Can you work these out from the model? Positions are in its coordinate system, mm. Coordinates: 2 decimals unless noted, no trailing zeros. Order: outer loops, then holes, each group sorted by start corner. A loop starts at its lowest first (then second) coordinate and runs counter-clockwise, first axis right, second up. Notation, with made-up numbers: (30.25, 10) -> (52.25, 10) arc R24 ccw to (52.25, 24) -> close; hole circle Ø3 at (89, -18). An arc over 180 degrees is marked (long way). Answer as a JSON object with one key per item and string values. Group by question number.
(1) I want a section at A-A, the plane x = -56. List the corners of the cut face in (y, z) for me, plus the area to 3 significant figures.
(2) If we mould it in two halves opening along X, with no side actions, what happens to faces 1 (the cylindrical face through (-65.287, 3.219, 9.248)), 2 (the flat face through (-1, 6.35, 0)), 3 (the cylindrical face through (-58.747, 3.131, -0.121))? For each: pulls with the +X half, pulls with the -X half, needs draft (parallel to the pull), parting line crosses it, or undercut.
(3) I want a section at B-B, the plane z = 0. List the corners of the cut face in (x, y) for me.
(4) I need wall thicknesses on line 1 (X direction, y = 1.75, z = 0); line 2 (Z direction, x = -56, y = 1.75); line 3 (X direction, y = 2.5, z = -2). Which ranges of each line are inside material? Lowest first, please.
(5) I want a section at C-C, the plane y = 4.75. List the corners of the cut face in (x, z) for me, plus the area to 3 significant figures.
from build123d import *

# Parameters (mm, degrees)
SKETCH1_W           = 132
SKETCH1_H           = 20
SKETCH1_R           = 2.75
BOSS_EXTRUDE1_DEPTH = 6.35
FILLET1_R           = 2.5


with BuildPart() as part:
    # Sketch1 → Boss-Extrude1 (new body)
    with BuildSketch(Plane(origin=(0, 0, 0), x_dir=(1, 0, 0), z_dir=(0, 1, 0))):
        Rectangle(SKETCH1_W, SKETCH1_H)
        with Locations((-56, 0)):
            Circle(SKETCH1_R, mode=Mode.SUBTRACT)
        with Locations((56, 0)):
            Circle(SKETCH1_R, mode=Mode.SUBTRACT)
    extrude(amount=BOSS_EXTRUDE1_DEPTH)

    # Fillet1
    fillet1_edges = [part.edges().sort_by_distance(p)[0] for p in [
        (-66, 3.175, -10),
        (66, 3.175, -10),
        (66, 3.175, 10),
        (-66, 3.175, 10),
    ]]
    fillet(fillet1_edges, radius=FILLET1_R)


solid = part.part
Computed values:
{
 "1": {"outline": "(0, -10) -> (6.35, -10) -> (6.35, -2.75) -> (0, -2.75) -> close; (0, 2.75) -> (6.35, 2.75) -> (6.35, 10) -> (0, 10) -> close", "area": "92.1 mm2"},
 "2": {"face 1": "pulls with the -X half", "face 2": "needs draft", "face 3": "undercut"},
 "3": {"outline": "(-66, 0) -> (-58.75, 0) -> (-58.75, 6.35) -> (-66, 6.35) -> close; (-53.25, 0) -> (53.25, 0) -> (53.25, 6.35) -> (-53.25, 6.35) -> close; (58.75, 0) -> (66, 0) -> (66, 6.35) -> (58.75, 6.35) -> close"},
 "4": {"line 1": "x = -66 to -58.75, -53.25 to 53.25, 58.75 to 66", "line 2": "z = -10 to -2.75, 2.75 to 10", "line 3": "x = -66 to -57.89, -54.11 to 54.11, 57.89 to 66"},
 "5": {"outline": "(-66, -7.5) arc R2.5 ccw to (-63.5, -10) -> (63.5, -10) arc R2.5 ccw to (66, -7.5) -> (66, 7.5) arc R2.5 ccw to (63.5, 10) -> (-63.5, 10) arc R2.5 ccw to (-66, 7.5) -> close; hole circle Ø5.5 at (-56, 0); hole circle Ø5.5 at (56, 0)", "area": "2,590 mm2"}
}
